Study the drawing (mm; zero at the part's minimum x, y, z) and answer. A direction names the side the tool comes from. Round coordinates to 2 decimals unless told otherwise and drop trailing zeros. Loops run counter-clockwise (first coordinate to the right, second up) from the corner with the lowest first, then second, coordinate; pieces in that order, holes last. Notation, with made-up numbers: M 73,-27 L 106,-27 A18 cw 106,-2 Z; hole C 7.5,80 d3. An arc over 180 degrees is marked long. Write each question's results on one line, items separated by ' | '.
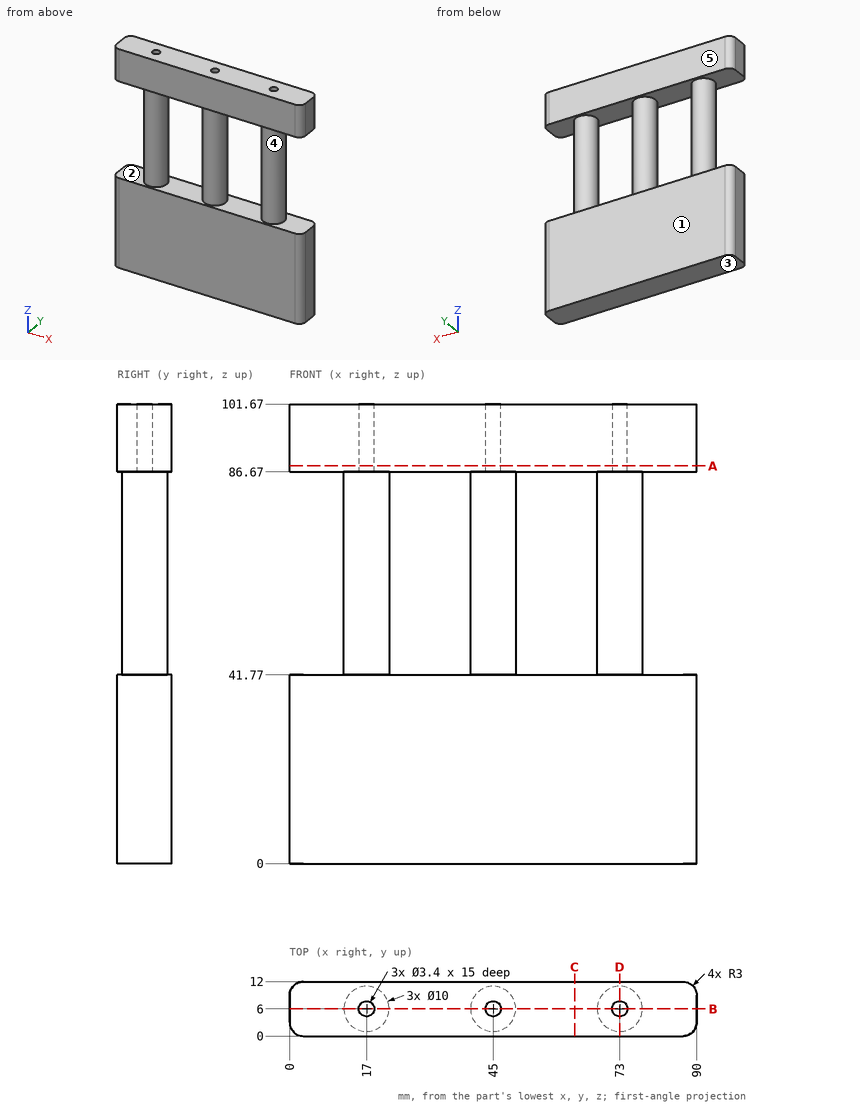
Item 1: The part is cut by section C-C (x = 63). Determine the outline of the cut face in (y, z), plus the area to 3 significant figures.
Outcome:
outline: M 0,0 L 12,0 L 12,41.77 L 0,41.77 Z; M 0,86.67 L 12,86.67 L 12,101.67 L 0,101.67 Z | area: 681 mm2
Item 2: The part is cut by section D-D (x = 73). Determine the outline of the cut face in (y, z), plus the area to 3 significant figures.
Outcome:
outline: M 0,0 L 12,0 L 12,41.77 L 11,41.77 L 11,86.67 L 12,86.67 L 12,101.67 L 7.7,101.67 L 7.7,86.67 L 4.3,86.67 L 4.3,101.67 L 0,101.67 L 0,86.67 L 1,86.67 L 1,41.77 L 0,41.77 Z | area: 1,080 mm2
Item 3: The mould has two halves that part along Z. Classify the marked faces 1, 2 and 3: pulls with the +Z half, pulls with the -Z half, needs draft (parallel to the pull), parting line crosses it, or undercut.
Outcome:
face 1: needs draft | face 2: undercut | face 3: pulls with the -Z half
Item 4: The part is cut by section A-A (z = 88). Determine the outline of the cut face in (x, y).
Outcome:
outline: M 0,3 A3 ccw 3,0 L 87,0 A3 ccw 90,3 L 90,9 A3 ccw 87,12 L 3,12 A3 ccw 0,9 Z; hole C 17,6 d3.4; hole C 45,6 d3.4; hole C 73,6 d3.4
Item 5: For the marked faces 4 and 5, determine the directions among +Z, -Z, +X, -X, +Y, -Y from which every point of the face is accessible in a straight line to the end or side of a thin tool.
Outcome:
face 4: none | face 5: +Z, -Z, +X, -X, +Y
Item 6: Straight lines are drawn through the part: line 1 (X direction, y = 6, z = 93.75); line 2 (Z direction, x = 67.5, y = 10); line 3 (Y direction, x = 17, z = 96.5). For each, find the intervals that lie inside material, in ascending order.
Outcome:
line 1: x = 0 to 15.3, 18.7 to 43.3, 46.7 to 71.3, 74.7 to 90 | line 2: z = 0 to 41.77, 86.67 to 101.67 | line 3: y = 0 to 4.3, 7.7 to 12
Item 7: The part is cut by section B-B (y = 6). State how many separate pieces and enclosed holes the cut face has, plus the area to 3 significant figures.
Outcome:
separate pieces: 1 | enclosed holes: 2 | area: 6,300 mm2
Item 8: A flat-ended cylindrical pin translates along its axis: pin 1 (3 mm diameter, centred on x = 17, y = 6, fed in from +Z). Find the tip coordinate at first contact, or state that the pin passes through.
Outcome:
pin 1: stops at z = 86.67
